Source: CAD feature listing. Evaluate the final solid. Frame: model axes, mm. A direction names the side the tool comes from. Give positions to 0.01 mm unless a question says otherwise; leave off trailing zeros. Loops run counter-clockwise (first coordinate to the right, second up) from the corner with the lowest first, then second, coordinate; pieces in that order, holes last. Notation, with made-up numbers: M 72,-39.5 L 120,-39.5 A23 cw 120,-19.5 Z; hole C 28.25,27.5 d3. An arc over 180 degrees is marked long. Write item = value, one per line.
Autodesk Inventor part; units mm, degrees
ref_plane "YZ Plane" through (0, 0, 0) normal (1, 0, 0) x (0, 1, 0)
ref_plane "XZ Plane" through (0, 0, 0) normal (0, 1, 0) x (-1, 0, 0)
ref_plane "XY Plane" through (0, 0, 0) normal (0, 0, 1) x (1, 0, 0)
sketch "Sketch1" plane through (0, 0, 0) normal (0, 0, 1) x (1, 0, 0)
  line L0 (0, -4.5) -> (-6, -4.5)
  line L1 (-6, -4.5) -> (-6, 11.5)
  line L2 (-6, 11.5) -> (0, 11.5)
  line L3 (0, 11.5) -> (0, -4.5)
  point P0 (0, 0)
  dimension "d0" = 6
  dimension "d1" = 16
  dimension "d17" = 0
  dimension "d18" = 11.5
extrude "Extrusion1" add sketch "Sketch1" along normal blind 3.9
sketch "Sketch2" plane through (-6, -4.5, 0) normal (0, -1, 0) x (1, 0, 0)
  point P0 (6, 0)
sketch "Sketch3" plane through (-6, -4.5, 0) normal (0, -1, 0) x (1, 0, 0)
  line L0 (0, 3.9) -> (6, 3.9)
  line L1 (6, 0) -> (6, 3.9)
  line L2 (0, 3.9) -> (6, 3.9)
  line L3 (6, 3.9) -> (6, 1.1)
  line L4 (6, 1.1) -> (0, 1.1)
  line L5 (0, 1.1) -> (0, 3.9)
  dimension "d4" = 2.8
extrude "Extrusion2" add sketch "Sketch3" along normal blind 9.9
sketch "Sketch4" plane through (0, 0, 3.9) normal (0, 0, 1) x (1, 0, 0)
  point P0 (0, 0)
  point P1 (-3, 8)
  point P2 (-3, 0)
hole "Hole1" at (-3, 8, 3.9) at (-3, 0, 3.9) direction (0, 0, -1) diameter 3 end through all
properties part number "GT2 belt clamp" material "Aluminum 6061"
1. Reachability of faces 4 (the flat face through (-3, 4, 0)), 5 (the flat face through (-3, -9, 1.1)) from +Z, -Z, +X, -X, +Y, -Y: full face, straight path, thin tool, end or side. Return the list, or none.
Derived:
face_4 = -Z, +X, -X, +Y, -Y
face_5 = -Z, +X, -X, -Y
2. Cut plane B-B, the plane y = 8. Return the cut outline in (x, z).
Derived:
outline = M -6,0 L -4.5,0 L -4.5,3.9 L -6,3.9 Z; M -1.5,0 L 0,0 L 0,3.9 L -1.5,3.9 Z
3. Cut plane D-D, the plane x = -5.55. Return the cut outline in (y, z), then the cut area to 3 significant figures.
Derived:
outline = M -14.4,1.1 L -4.5,1.1 L -4.5,0 L 11.5,0 L 11.5,3.9 L -14.4,3.9 Z
area = 90.1 mm²
4. Cut plane C-C, the plane z = 0.45. Return the cut outline in (x, y).
Derived:
outline = M -6,-4.5 L 0,-4.5 L 0,11.5 L -6,11.5 Z; hole C -3,0 d3; hole C -3,8 d3
5. First-contact query: pin 1 Ø0.6 at (x, z) = (-2, 0.5) entering from -Y; pin 2 Ø3 at (x, y) = (-4.5, -11) entering from -Z. Flat tips, straight axial feed; report the tip coordinate or a pass-through.
Derived:
pin_1 = -4.5
pin_2 = 1.1
6. Cut plane A-A, the plane x = -3. Return the cut outline in (y, z).
Derived:
outline = M -14.4,1.1 L -4.5,1.1 L -4.5,0 L -1.5,0 L -1.5,3.9 L -14.4,3.9 Z; M 1.5,0 L 6.5,0 L 6.5,3.9 L 1.5,3.9 Z; M 9.5,0 L 11.5,0 L 11.5,3.9 L 9.5,3.9 Z
7. Material intervals for probe 1 along Y at (x, z) = (-3, 2); probe 2 along Y at (x, z) = (-3, 0.9); probe 3 along X at (y, z) = (0, 1.05), sorted ascending. Write a range as from..to.
Derived:
probe_1 = -14.4..-1.5, 1.5..6.5, 9.5..11.5
probe_2 = -4.5..-1.5, 1.5..6.5, 9.5..11.5
probe_3 = -6..-4.5, -1.5..0
8. Pull-direction query (X, two-part tool) for faces 1 (the flat face through (-6, -2, 2)), 2 (the flat face through (0, -1, 2)), 3 (the cylindrical face through (-1.536, 0.325, 1.923)); classes: +X half, -X half, draft (parallel to the pull), parting line (faces both ways), or undercut.
Derived:
face_1 = -X half
face_2 = +X half
face_3 = undercut
